from build123d import *

# Parameters (mm, degrees)
ESQUISSE1_R                  = 1.5
BOSS_EXTRU_1_DEPTH           = 8
CONG_1_R                     = 8
ESQUISSE2_W                  = 20.5
ESQUISSE2_H                  = 8.937448888
ENL_V_MAT_EXTRU_1_DEPTH      = 10
ENL_V_MAT_EXTRU_2_DEPTH      = 5
ESQUISSE4_W                  = 5.650854606
ESQUISSE4_H                  = 10
ENL_V_MAT_EXTRU_3_DEPTH      = 5
ENL_V_MAT_EXTRU_4_DEPTH      = 40.644055588
ENL_V_MAT_EXTRU_4_DEPTH_BACK = 40.644055588
ESQUISSE6_R                  = 1.5
ENL_V_MAT_EXTRU_5_REACH      = 37.743
ESQUISSE7_W                  = 20.5
ESQUISSE7_H                  = 5.5
CHANFREIN1_SIZE2             = 1.5
CHANFREIN1_SIZE              = 5.5
CONG_2_R                     = 3


with BuildPart() as part:
    # Esquisse1 → Boss.-Extru.1 (new, symmetric)
    with BuildSketch(Plane.XY):
        with BuildLine():
            Line((15, 0), (-15, 0))
            Line((-15, 0), (-18.52357943, 18.05834458))
            ThreePointArc((-18.52357943, 18.05834458), (-18.248833113, 20.232434219), (-16.735143225, 21.817014359))
            ThreePointArc((-16.735143225, 21.817014359), (0, 26), (16.735143225, 21.817014359))
            ThreePointArc((16.735143225, 21.817014359), (18.248833113, 20.232434219), (18.52357943, 18.05834458))
            Line((18.52357943, 18.05834458), (15, 0))
        make_face()
        with Locations((-14, 19.25)):
            Circle(ESQUISSE1_R, mode=Mode.SUBTRACT)
        with Locations(Location((14, 19.25, 0), (0, 0, 180))):
            Circle(ESQUISSE1_R, mode=Mode.SUBTRACT)
    extrude(amount=BOSS_EXTRU_1_DEPTH, both=True)

    # Congé1
    cong_1_edges = [part.edges().sort_by_distance(p)[0] for p in [
        (0, 0, -8),
        (0, 0, 8),
    ]]
    fillet(cong_1_edges, radius=CONG_1_R - 0.0001)  # a hair under: the kernel refuses the full size

    # Esquisse2 → Enlèv. mat.-Extru.1 (cut, symmetric)
    with BuildSketch(Plane.XY):
        with Locations((0, 3.531275556)):
            Rectangle(ESQUISSE2_W, ESQUISSE2_H)
    extrude(amount=ENL_V_MAT_EXTRU_1_DEPTH, both=True, mode=Mode.SUBTRACT)

    # Esquisse3 → Enlèv. mat.-Extru.2 (cut, symmetric)
    with BuildSketch(Plane.XY):
        with BuildLine():
            Line((7, 25.304379858), (4.599145394, 13))
            Line((4.599145394, 13), (17.536585366, 13))
            Line((17.536585366, 13), (18.52357943, 18.05834458))
            ThreePointArc((18.52357943, 18.05834458), (18.248833113, 20.232434219), (16.735143225, 21.817014359))
            ThreePointArc((16.735143225, 21.817014359), (11.994985849, 23.916379883), (7, 25.304379858))
        make_face()
        with BuildLine():
            Line((-17.536585366, 13), (-18.52357943, 18.05834458))
            ThreePointArc((-18.52357943, 18.05834458), (-18.248833113, 20.232434219), (-16.735143225, 21.817014359))
            ThreePointArc((-16.735143225, 21.817014359), (-11.994985849, 23.916379883), (-7, 25.304379858))
            Line((-7, 25.304379858), (-4.599145394, 13))
            Line((-4.599145394, 13), (-17.536585366, 13))
        make_face()
    extrude(amount=ENL_V_MAT_EXTRU_2_DEPTH, both=True, mode=Mode.SUBTRACT)

    # Esquisse4 → Enlèv. mat.-Extru.3 (cut)
    with BuildSketch(Plane(origin=(0, 13, 0), x_dir=(1, 0, 0), z_dir=(0, 1, 0))):
        with Locations((7.424572697, 0)):
            Rectangle(ESQUISSE4_W, ESQUISSE4_H)
        with Locations((-7.424572697, 0)):
            Rectangle(ESQUISSE4_W, ESQUISSE4_H)
    extrude(amount=-ENL_V_MAT_EXTRU_3_DEPTH, mode=Mode.SUBTRACT)

    # Esquisse6 → Enlèv. mat.-Extru.4 (cut, two sides: drawn at the far end of the back side and taken through both)
    with BuildSketch(Plane.ZY.offset(-10.25).offset(-ENL_V_MAT_EXTRU_4_DEPTH_BACK)):
        with Locations(Location((0, 8, 0), (0, 0, 270))):
            Circle(ESQUISSE6_R)
    extrude(amount=ENL_V_MAT_EXTRU_4_DEPTH + ENL_V_MAT_EXTRU_4_DEPTH_BACK, mode=Mode.SUBTRACT)

    # Enlèv. mat.-Extru.5: up to this face of the body (flat: up to its plane)
    enl_v_mat_extru_5_end = Plane(part.part.faces().sort_by_distance((10.657947806, 16.753093671, 5))[0])
    # Esquisse7 → Enlèv. mat.-Extru.5 (cut, up to the picked face)
    with BuildSketch(Plane(origin=(0, 0, -8), x_dir=(-1, 0, 0), z_dir=(0, 0, -1)), mode=Mode.PRIVATE) as enl_v_mat_extru_5_sk1:
        with Locations((0, 10.75)):
            Rectangle(ESQUISSE7_W, ESQUISSE7_H)
    enl_v_mat_extru_5_tool1 = split(extrude(enl_v_mat_extru_5_sk1.sketch, amount=-ENL_V_MAT_EXTRU_5_REACH, mode=Mode.PRIVATE), bisect_by=enl_v_mat_extru_5_end, keep=Keep.BOTH, mode=Mode.PRIVATE)
    add(enl_v_mat_extru_5_tool1.solids().sort_by(Axis((0, 10.75, -8), (0, 0, 1)))[0], mode=Mode.SUBTRACT)

    # Chanfrein1
    chanfrein1_edges = [part.edges().sort_by_distance(p)[0] for p in [
        (0, 8, 5),
    ]]
    chanfrein1_side = [part.faces().sort_by_distance(p)[0] for p in [
        (0, 8.03, 5),
    ]]
    chamfer(chanfrein1_edges, length=CHANFREIN1_SIZE - 0.0001, length2=CHANFREIN1_SIZE2 - 0.0001, reference=chanfrein1_side[0])  # a hair under: the kernel refuses the full size

    # Congé2
    cong_2_edges = [part.edges().sort_by_distance(p)[0] for p in [
        (7, 25.304379858, 0),
        (-7, 25.304379858, 0),
    ]]
    fillet(cong_2_edges, radius=CONG_2_R)


solid = part.part
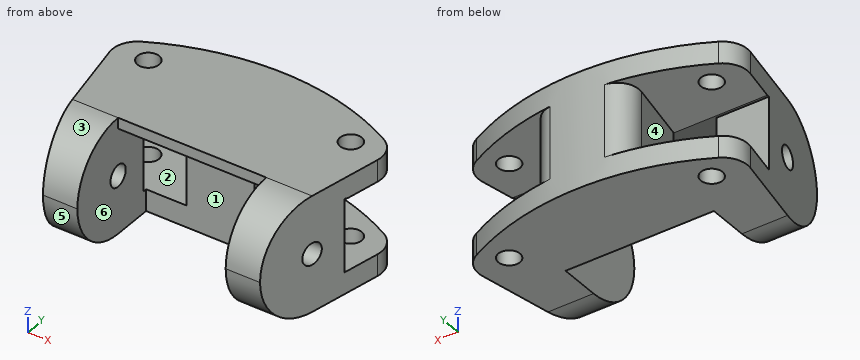
The listing builds one solid part. Answer for the finished solid, in the listing's coordinates (mm). Face numbers are marked on the shaded views. A direction names the side the tool comes from. Coordinates: 2 decimals unless noted, no trailing zeros. Loops run counter-clockwise (first coordinate to the right, second up) from the corner with the lowest first, then second, coordinate; pieces in that order, holes last. Notation, with made-up numbers: M 60.5,82 L 88.5,82 A21 cw 88.5,112 Z; hole C 5.5,4.5 d7. An arc over 180 degrees is marked long. Answer in a Markdown table with one row per item.
1) Find section B-B (z = 2.75). Determine the outline of the cut face in (x, y), then the cut area to 3 significant figures.
Answers below:
| item | result |
|---|---|
| outline | M -17.54,13 L -15.1,0.49 L -10.25,0.49 L -10.25,13 Z; M -6.4,22.24 L -4.7,13.5 L 4.7,13.5 L 6.4,22.24 A3 ccw 3.78,25.8 A35.57 ccw -3.78,25.8 A3 ccw Z; M 10.25,0.49 L 15.1,0.49 L 17.54,13 L 10.25,13 Z |
| area | 292 mm^2 |
2) Find the intervals of material crossed by probe 1 along Z at (x, y) = (-6.5, 17.25); probe 2 along Z at (x, y) = (-13.5, 8); probe 3 along Y at (x, z) = (-11.75, 0), in increasing order.
Answers below:
| item | result |
|---|---|
| probe 1 | -8 to -5, 5 to 8 |
| probe 2 | -8 to -1.5, 1.5 to 8 |
| probe 3 | 0 to 6.5, 9.5 to 13 |
3) Find section C-C (y = 2.5). Determine the outline of the cut face in (x, z), then the cut area to 3 significant figures.
Answers below:
| item | result |
|---|---|
| outline | M -15.49,-5.81 L -10.25,-5.81 L -10.25,5.81 L -15.49,5.81 Z; M 10.25,-5.81 L 15.49,-5.81 L 15.49,5.81 L 10.25,5.81 Z |
| area | 122 mm^2 |
4) Which of the six approach directions +Z, -Z, +X, -X, +Y, -Y give full straight-line access (tool end or side, diameter ignored) to the marked faces 4, 5 and 6?
Answers below:
| item | result |
|---|---|
| face 4 | -X, -Y |
| face 5 | -Z, +X, -X, -Y |
| face 6 | -Z, -Y |
5) Determine the mould class of the marked faces 1, 2 and 3 for opening direction Z: released by +Z, released by -Z, zero draft, split by the parting line, or undercut.
Answers below:
| item | result |
|---|---|
| face 1 | zero draft |
| face 2 | undercut |
| face 3 | released by +Z |
6) Given pin 1 (10 mm diameter, centred on x = -6, y = 9, fed in from -Z); pin 2 (4 mm diameter, centred on x = -2, z = 1, fed in from -Y); pin 3 (3 mm diameter, centred on x = 12.5, z = 5.5, fed in from +Y); pin 4 (1.7 mm diameter, centred on x = 2.5, z = 7, fed in from -Y), each flat-ended and moving along its own axis, determine where each tip first touches the part or whether it passes through.
Answers below:
| item | result |
|---|---|
| pin 1 | z = -8 |
| pin 2 | y = 13.5 |
| pin 3 | y = 24.26 |
| pin 4 | y = 8 |
7) Find section D-D (x = -8). Determine the outline of the cut face in (y, z), then the cut area to 3 significant figures.
Answers below:
| item | result |
|---|---|
| outline | M 8,6.5 L 13.5,5 L 25.09,5 L 25.09,8 L 8,8 Z; M 13.5,-8 L 25.09,-8 L 25.09,-5 L 13.5,-5 Z |
| area | 81.9 mm^2 |
8) Find section A-A (x = 14). Count the separate pieces of the cut face and the enclosed holes in it, then the cut area to 3 significant figures.
Answers below:
| item | result |
|---|---|
| separate pieces | 3 |
| enclosed holes | 1 |
| area | 216 mm^2 |
